Verification items for the finished model (mm, model axes). Coordinates: 2 decimals unless noted, no trailing zeros. Order: outer loops, then holes, each group sorted by start corner. A loop starts at its lowest first (then second) coordinate and runs counter-clockwise, first axis right, second up. Notation, with made-up numbers: M 56.25,65 L 77.25,65 A18 cw 77.25,74 Z; hole C -28,-18.5 d3. An arc over 180 degrees is marked long. Return JSON: item names as keys, results as strings. Group by question number.
Q1. Section check B-B, the plane y = 30.5. Enter the section's corners in (x, z), then the cut area to 3 significant figures.
Q2. Section check A-A, the plane z = 0.45. Enter the section's corners in (x, y).
Q3. Thickness scan on probe 1 along X at (y, z) = (-42, 2.3); probe 2 along X at (y, z) = (-7, 1.85); probe 3 along X at (y, z) = (14.5, 1.2). Record the ranges inside material, lowest first.
Q4. Mould release check, pull along Y, two halves, no side actions. Record for faces 1 (the face through (-72.8, -43.61, 1.37)), 2 (the face through (-1, 1, 0)), 3 (the face through (68.95, -55.04, 1.33)): pulls with the +Y half, pulls with the -Y half, needs draft (parallel to the pull), parting line crosses it, or undercut.
Q5. Section check C-C, the plane x = 70. Enter the section's corners in (y, z), then the cut area to 3 significant figures.
from build123d import *

# Parameters (mm, degrees)
Y_KSEKLIK_EKSTR_ZYON3_DEPTH = 2.7
IZIM2_R                     = 3.79
KES_EKSTR_ZYON1_DEPTH       = 2.75


with BuildPart() as part:
    # Çizim1 → Yükseklik-Ekstrüzyon3 (new body)
    with BuildSketch(Plane.XY):
        with BuildLine():
            Line((-90, -75), (20, -75))
            ThreePointArc((20, -75), (69.497474683, -54.497474683), (90, -5))
            Line((90, -5), (90, 5))
            ThreePointArc((90, 5), (69.497474683, 54.497474683), (20, 75))
            Line((20, 75), (-90, 75))
            Line((-90, 75), (-90, -75))
        make_face()
    extrude(amount=Y_KSEKLIK_EKSTR_ZYON3_DEPTH)

    # Çizim2 → Kes-Ekstrüzyon1 (cut)
    with BuildSketch(Plane.XY.offset(2.7)):
        with Locations((-69.187191481, 42.468560625)):
            Circle(IZIM2_R)
        with Locations((20.812808519, 42.468560625)):
            Circle(IZIM2_R)
        with Locations(Location((20.812808519, -42.468560625, 0), (0, 0, 180))):
            Circle(IZIM2_R)
        with Locations(Location((-69.187191481, -42.468560625, 0), (0, 0, 180))):
            Circle(IZIM2_R)
    extrude(amount=-KES_EKSTR_ZYON1_DEPTH, mode=Mode.SUBTRACT)


solid = part.part
Numbers:
{
 "1": {"outline": "M -90,0 L 85.19,0 L 85.19,2.7 L -90,2.7 Z", "area": "473 mm2"},
 "2": {"outline": "M -90,-75 L 20,-75 A70 ccw 90,-5 L 90,5 A70 ccw 20,75 L -90,75 Z; hole C -69.19,-42.47 d7.58; hole C -69.19,42.47 d7.58; hole C 20.81,-42.47 d7.58; hole C 20.81,42.47 d7.58"},
 "3": {"probe 1": "x = -90 to -72.95, -65.43 to 17.05, 24.57 to 79.42", "probe 2": "x = -90 to 89.97", "probe 3": "x = -90 to 89.35"},
 "4": {"face 1": "undercut", "face 2": "needs draft", "face 3": "pulls with the -Y half"},
 "5": {"outline": "M -53.99,0 L 53.99,0 L 53.99,2.7 L -53.99,2.7 Z", "area": "292 mm2"}
}
